Check sheet for the modelled part. Datum: model origin and axes. Units: mm. A direction names the side the tool comes from. Round coordinates to 2 decimals unless told otherwise and drop trailing zeros. Write each loop counter-clockwise with the first axis right and the second up, starting at its lowest first coordinate (ties: lowest second). Pieces come first, ordered by that corner, then holes. Notation, with made-up numbers: (0, 61.5) -> (22, 61.5) arc R26 cw to (22, 99.5) -> close; hole circle Ø8 at (11, -18.5). An arc over 180 degrees is marked (long way). One line per item, written item: value.
from build123d import *

# Parameters (mm, degrees)
BOSS_EXTRU_1_DEPTH      = 30
ESQUISSE3_R             = 2.6
ENL_V_MAT_EXTRU_1_DEPTH = 6
CHANFREIN1_SIZE         = 1


with BuildPart() as part:
    # Esquisse1 → Boss.-Extru.1 (new body)
    with BuildSketch(Plane.XY):
        with BuildLine():
            Line((-27.6, 0), (-17.6, 0))
            ThreePointArc((-17.6, 0), (0, 17.6), (17.6, 0))
            Line((17.6, 0), (27.6, 0))
            Line((27.6, 0), (27.6, -5))
            Line((27.6, -5), (10.3, -5))
            Line((10.3, -5), (10.3, 0))
            ThreePointArc((10.3, 0), (0, 10.3), (-10.3, 0))
            Line((-10.3, 0), (-10.3, -5))
            Line((-10.3, -5), (-27.6, -5))
            Line((-27.6, -5), (-27.6, 0))
        make_face()
    extrude(amount=BOSS_EXTRU_1_DEPTH)

    # Esquisse3 → Enlèv. mat.-Extru.1 (cut, through all)
    with BuildSketch(Plane(origin=(0, 0, 0), x_dir=(1, 0, 0), z_dir=(0, 1, 0))):
        with Locations((-22.6, -15)):
            Circle(ESQUISSE3_R)
        with Locations((22.6, -15)):
            Circle(ESQUISSE3_R)
    extrude(amount=-ENL_V_MAT_EXTRU_1_DEPTH, mode=Mode.SUBTRACT)

    # Chanfrein1
    chanfrein1_edges = [part.edges().sort_by_distance(p)[0] for p in [
        (-10.3, -5, 15),
        (10.3, -5, 15),
    ]]
    chamfer(chanfrein1_edges, length=CHANFREIN1_SIZE)


solid = part.part
Item 1: Sectioned sample at D-D on z = 22. Enter the section's corners in (x, y), and give its area (3 significant figures).
Answer:
outline: (-27.6, -5) -> (-11.3, -5) -> (-10.3, -4) -> (-10.3, 0) arc R10.3 cw to (10.3, 0) -> (10.3, -4) -> (11.3, -5) -> (27.6, -5) -> (27.6, 0) -> (17.6, 0) arc R17.6 ccw to (-17.6, 0) -> (-27.6, 0) -> close
area: 492 mm^2
Item 2: Sectioned sample at A-A on z = 15. Enter the section's corners in (x, y).
Answer:
outline: (-27.6, -5) -> (-25.2, -5) -> (-25.2, 0) -> (-27.6, 0) -> close; (-20, -5) -> (-11.3, -5) -> (-10.3, -4) -> (-10.3, 0) arc R10.3 cw to (10.3, 0) -> (10.3, -4) -> (11.3, -5) -> (20, -5) -> (20, 0) -> (17.6, 0) arc R17.6 ccw to (-17.6, 0) -> (-20, 0) -> close; (25.2, -5) -> (27.6, -5) -> (27.6, 0) -> (25.2, 0) -> close
Item 3: Sectioned sample at B-B on x = 22.6. Enter the section's corners in (y, z), and give its area (3 significant figures).
Answer:
outline: (-5, 0) -> (0, 0) -> (0, 12.4) -> (-5, 12.4) -> close; (-5, 17.6) -> (0, 17.6) -> (0, 30) -> (-5, 30) -> close
area: 124 mm^2
Item 4: Thickness scan on line 1 (X direction, y = -2.85, z = 15); line 2 (Z direction, x = -22.6, y = -1.55); line 3 (X direction, y = -3.5, z = 9). Record the ranges inside material, lowest first.
Answer:
line 1: x = -27.6 to -25.2, -20 to -10.3, 10.3 to 20, 25.2 to 27.6
line 2: z = 0 to 12.4, 17.6 to 30
line 3: x = -27.6 to -10.3, 10.3 to 27.6
Item 5: Tool access check on faces 1 (the cylindrical face through (-24.663, -2.465, 16.582)), 2 (the flat face through (19, 0, 15)), 3 (the flat face through (19.6, -5, 14.8)), 4 (the flat face through (-10.3, -2, 15)), 5 (the flat face through (-19, 0, 15)). Record the directions out of +Z, -Z, +X, -X, +Y, -Y that give a thin tool (end or side, any length) a straight path to the whole face; none if there is none.
Answer:
face 1: +Y, -Y
face 2: +Z, -Z, +X, +Y
face 3: +Z, -Z, +X, -X, -Y
face 4: +Z, -Z, -Y
face 5: +Z, -Z, -X, +Y
Item 6: Sectioned sample at C-C on y = 4. Enter the section's corners in (x, z).
Answer:
outline: (-17.14, 0) -> (-9.49, 0) -> (-9.49, 30) -> (-17.14, 30) -> close; (9.49, 0) -> (17.14, 0) -> (17.14, 30) -> (9.49, 30) -> close
Item 7: Depth check by flat-ended pin: P1, Ø8.5, axis at x = 22.6, z = 15, coming from the +Y side; P2, Ø5, axis at y = 14, z = 6.5, coming from the -X side; P3, Ø3, axis at x = -1.5, z = 23.5, coming from the -Y side. Enter the tip coordinate at first touch or a pass-through.
Answer:
P1: stops at y = 0
P2: stops at x = -13.32
P3: stops at y = 9.85
